Part model, mm, in its own coordinate system. A direction names the side the tool comes from. Round coordinates to 2 decimals unless told otherwise and drop trailing zeros. Order: outer loops, then holes, each group sorted by start corner. A loop starts at its lowest first (then second) coordinate and runs counter-clockwise, first axis right, second up. Notation, with made-up numbers: M -31,-5 L -2,-5 A20 ccw -2,22 Z; hole C 0.25,85 d3. An arc over 180 degrees is marked long. Write each question's results on one line, items separated by ' | '. Start each with the question number.
1. Which spindle directions (+Z, -Z, +X, -X, +Y, -Y) get a long thin tool onto all of the face, cutting with end or side? Do faces 1 (the face through (2.146, -21.579, 4.676)), 2 (the face through (-2.5, -13, -5)), 3 (the face through (0, -21, 7.5)). Say none if no direction does.
2. Probe L1, parallel to X at y = -21.25, z = 4; L2, parallel to Z at x = 0, y = -20.75; L3, parallel to Y at x = 1.75, z = 4. List the from-to ranges inside material, lowest first. Write a range as [from, to].
3. Two-plate mould, pull along Z, no slides. Class faces 4 (the face through (-9.965, -13.405, -3.896)), 5 (the face through (-12.5, -12, -5)), 6 (the face through (-5, -12, -7.5)), 7 (the face through (0.105, -12.684, -1.997)): +Z half, -Z half, draft (parallel to the pull), parting line (faces both ways), or undercut.
4. Band-saw the part on C-C, the plane y = -12.5. List the corners of the cut face in (x, z), then the cut area to 3 significant figures.
5. Band-saw the part on A-A, the plane x = 0. List the corners of the cut face in (y, z), then the cut area to 3 significant figures.
6. Drop a flat-ended pin along its axis: pin 1 Ø10 at (x, y) = (-6, -11) entering from +Z. Give the stop position or say it passes through.
7. Band-saw the part on D-D, the plane z = -5.75. List the corners of the cut face in (x, y).
8. Band-saw the part on B-B, the plane z = 4. List the corners of the cut face in (x, y), then the cut area to 3 significant figures.
```python
from build123d import *

# Parameters (mm, degrees)
F0_W     = 15
F0_H     = 15
F1_DEPTH = 25
F2_W     = 5
F2_H     = 5
F3_DEPTH = 25
F5_D     = 12
F6_R     = 1.6830383024
F7_DEPTH = 5
F8_R     = 2.25
F9_DEPTH = 6.9388512347


with BuildPart() as f1:
    # F0 (on Front) → F1 (new body)
    with BuildSketch(Plane.XZ):
        Rectangle(F0_W, F0_H)
    extrude(amount=F1_DEPTH)

    # F2 (on face) → F3 (cut)
    with BuildSketch(Plane.XZ.offset(25)):
        with Locations((0, -5)):
            Rectangle(F2_W, F2_H)
    extrude(amount=-F3_DEPTH, mode=Mode.SUBTRACT)

    # F5 (through all)
    with Locations(Plane(origin=(-7.5, 0, 0), x_dir=(0, -1, 0), z_dir=(-1, 0, 0))):
        with Locations((12.5, 4)):
            Hole(F5_D / 2)

    # F6 (on face) → F7 (join)
    with BuildSketch(Plane(origin=(-7.5, 0, 0), x_dir=(0, -1, 0), z_dir=(-1, 0, 0))):
        with Locations((12.5, -5.3153163753)):
            Circle(F6_R)
    extrude(amount=F7_DEPTH)

    # F8 (on face) → F9 (cut, through all)
    with BuildSketch(Plane.XZ.offset(25)):
        with Locations((0, 4)):
            Circle(F8_R)
    extrude(amount=-F9_DEPTH, mode=Mode.SUBTRACT)


solid = f1.part
```
Solution:
1) face 1: -Y | face 2: -Z, +Y, -Y | face 3: +Z, +X, -X, +Y, -Y
2) L1: [-7.5, -2.25], [2.25, 7.5] | L2: [-2.5, 1.75], [6.25, 7.5] | L3: [-6.5, 0]
3) face 4: parting line | face 5: draft | face 6: -Z half | face 7: undercut
4) outline: M -12.5,-7 L -7.5,-7 L -7.5,-7.5 L -2.5,-7.5 L -2.5,-2.5 L 2.5,-2.5 L 2.5,-7.5 L 7.5,-7.5 L 7.5,-2 L -7.5,-2 L -7.5,-3.63 L -12.5,-3.63 Z | area: 74.3 mm^2
5) outline: M -25,-2.5 L 0,-2.5 L 0,7.5 L -7.63,7.5 A6 cw long -18.06,1.75 L -25,1.75 Z; M -25,6.25 L -18.06,6.25 A6 cw -17.37,7.5 L -25,7.5 Z | area: 124 mm^2
6) pin 1: z = 7.5
7) outline: M -12.5,-14.13 L -7.5,-14.13 L -7.5,-25 L -2.5,-25 L -2.5,0 L -7.5,0 L -7.5,-10.87 L -12.5,-10.87 Z; M 2.5,-25 L 7.5,-25 L 7.5,0 L 2.5,0 Z
8) outline: M -7.5,-25 L -2.25,-25 L -2.25,-18.5 L -7.5,-18.5 Z; M -7.5,-6.5 L 7.5,-6.5 L 7.5,0 L -7.5,0 Z; M 2.25,-25 L 7.5,-25 L 7.5,-18.5 L 2.25,-18.5 Z | area: 166 mm^2
